```python
from build123d import *

# Parameters (mm, degrees)
F1_DEPTH  = 2
F2_DEPTH  = 10
F3_R      = 4
F4_DEPTH  = 10.001
F3_R_2    = 11
F5_DEPTH  = 8
F6_R      = 4
F7_DEPTH  = 10.001
F6_R_2    = 11
F8_DEPTH  = 8
F10_DEPTH = 8


with BuildPart() as f1:
    # F0 (on Top) → F1 (new body)
    with BuildSketch(Plane.XY):
        with BuildLine():
            ThreePointArc((12, 5), (11.7240041235, 2.4411472664), (10.9087121146, 0))
            Line((10.9087121146, 0), (69.0912878854, 0))
            ThreePointArc((69.0912878854, 0), (68, 5), (69.0912878854, 10))
            Line((69.0912878854, 10), (10.9087121146, 10))
            ThreePointArc((10.9087121146, 10), (11.7240041235, 7.5588527336), (12, 5))
        make_face()
    extrude(amount=F1_DEPTH)

    # F0 (on Top) → F2 (join)
    with BuildSketch(Plane.XY):
        with BuildLine():
            Line((10.9087121146, 0), (0, 0))
            Line((0, 0), (0, 10))
            Line((0, 10), (10.9087121146, 10))
            ThreePointArc((10.9087121146, 10), (-12, 5), (10.9087121146, 0))
        make_face()
        with BuildLine():
            ThreePointArc((69.0912878854, 10), (68, 5), (69.0912878854, 0))
            Line((69.0912878854, 0), (80, 0))
            Line((80, 0), (80, 10))
            Line((80, 10), (69.0912878854, 10))
        make_face()
        with BuildLine():
            Line((80, 0), (69.0912878854, 0))
            ThreePointArc((69.0912878854, 0), (82.5588527336, -6.7240041235), (92, 5))
            ThreePointArc((92, 5), (82.5588527336, 16.7240041235), (69.0912878854, 10))
            Line((69.0912878854, 10), (80, 10))
            Line((80, 10), (80, 0))
        make_face()
        with BuildLine():
            Line((0, 10), (0, 0))
            Line((0, 0), (10.9087121146, 0))
            ThreePointArc((10.9087121146, 0), (11.7240041235, 2.4411472664), (12, 5))
            ThreePointArc((12, 5), (11.7240041235, 7.5588527336), (10.9087121146, 10))
            Line((10.9087121146, 10), (0, 10))
        make_face()
    extrude(amount=F2_DEPTH)

    # F3 (on face) → F4 (cut, through all)
    with BuildSketch(Plane.XY.offset(10)):
        with Locations((0, 5)):
            Circle(F3_R)
    extrude(amount=-F4_DEPTH, mode=Mode.SUBTRACT)

    # F3 (on face) → F5 (cut)
    with BuildSketch(Plane.XY.offset(10)):
        with Locations((0, 5)):
            Circle(F3_R_2)
        with Locations((0, 5)):
            Circle(F3_R, mode=Mode.SUBTRACT)
    extrude(amount=-F5_DEPTH, mode=Mode.SUBTRACT)

    # F6 (on face) → F7 (cut, through all)
    with BuildSketch(Plane.XY.offset(10)):
        with Locations((80, 5)):
            Circle(F6_R)
    extrude(amount=-F7_DEPTH, mode=Mode.SUBTRACT)

    # F6 (on face) → F8 (cut)
    with BuildSketch(Plane.XY.offset(10)):
        with Locations((80, 5)):
            Circle(F6_R_2)
        with Locations((80, 5)):
            Circle(F6_R, mode=Mode.SUBTRACT)
    extrude(amount=-F8_DEPTH, mode=Mode.SUBTRACT)

    # F9 (on face) → F10 (join)
    with BuildSketch(Plane.XY.offset(2)):
        with BuildLine():
            ThreePointArc((10.9087121146, 10), (11.3081338214, 9.0157327447), (11.6189500386, 8))
            Line((11.6189500386, 8), (68.3810499614, 8))
            ThreePointArc((68.3810499614, 8), (68.6918661786, 9.0157327447), (69.0912878854, 10))
            Line((69.0912878854, 10), (10.9087121146, 10))
        make_face()
        with BuildLine():
            ThreePointArc((11.6189500386, 2), (11.3081338214, 0.9842672553), (10.9087121146, 0))
            Line((10.9087121146, 0), (69.0912878854, 0))
            ThreePointArc((69.0912878854, 0), (68.6918661786, 0.9842672553), (68.3810499614, 2))
            Line((68.3810499614, 2), (11.6189500386, 2))
        make_face()
    extrude(amount=F10_DEPTH)


solid = f1.part
```
The listing builds one solid part. Answer for the finished solid, in the listing's coordinates (mm). A direction names the side the tool comes from. Coordinates: 2 decimals unless noted, no trailing zeros. Write each loop counter-clockwise with the first axis right and the second up, starting at its lowest first coordinate (ties: lowest second). Pieces come first, ordered by that corner, then holes.
Q1. Section D-D, the plane x = 18 is taken. Write down the section's boundary in (y, z).
Returned:
outline: (0, 0) - (10, 0) - (10, 10) - (8, 10) - (8, 2) - (2, 2) - (2, 10) - (0, 10) - close
Q2. The mould has two halves that part along X. Classify faces 4 (the flat face through (40, 0, 5)), 5 (the flat face through (0, 0, 2)), 6 (the flat face through (40, 9, 10)): released by +X, released by -X, zero draft, split by the parting line, or undercut.
Returned:
face 4: undercut
face 5: undercut
face 6: zero draft
Q3. Find the intervals of material crossed by line 1 along Y through (x, z) = (0, 7); line 2 along Y through (x, z) = (0, 1.1); line 3 along X through (y, z) = (3.25, 4.25), in increasing order.
Returned:
line 1: y = -7 to -6, 16 to 17
line 2: y = -7 to 1, 9 to 17
line 3: x = -11.87 to -10.86, 10.86 to 11.87, 68.13 to 69.14, 90.86 to 91.87
Q4. Section C-C, the plane y = -1.25 is taken. Write down the section's boundary in (x, z), then the cut area to 3 significant figures.
Returned:
outline: (-10.24, 0) - (10.24, 0) - (10.24, 10) - (9.05, 10) - (9.05, 2) - (-9.05, 2) - (-9.05, 10) - (-10.24, 10) - close; (69.76, 0) - (90.24, 0) - (90.24, 10) - (89.05, 10) - (89.05, 2) - (70.95, 2) - (70.95, 10) - (69.76, 10) - close
area: 120 mm2
Q5. Given P1, Ø5, axis at y = 2, z = 4.5, coming from the -X side; P2, Ø4, axis at y = 14, z = 6.5, coming from the +X side; P3, Ø11, axis at x = -2.5, y = 8, coming from the +Z side, each flat-ended and moving along its own axis, determine where each tip first touches the part or whether it passes through.
Returned:
P1: stops at x = -11.99
P2: stops at x = 89.75
P3: stops at z = 2
Q6. Section A-A, the plane z = 4.25 is taken. Write down the section's boundary in (x, y).
Returned:
outline: (10.91, 0) - (69.09, 0) arc R12 ccw (long way) to (69.09, 10) - (10.91, 10) arc R12 ccw (long way) to start; hole circle Ø22 at (0, 5); hole (11.62, 2) - (68.38, 2) arc R12 cw to (68.38, 8) - (11.62, 8) arc R12 cw to start; hole circle Ø22 at (80, 5)
Q7. Section B-B, the plane x = 0 is taken. Write down the section's boundary in (y, z).
Returned:
outline: (-7, 0) - (1, 0) - (1, 2) - (-6, 2) - (-6, 10) - (-7, 10) - close; (9, 0) - (17, 0) - (17, 10) - (16, 10) - (16, 2) - (9, 2) - close
Q8. Which of the six approach directions +Z, -Z, +X, -X, +Y, -Y give full straight-line access (tool end or side, diameter ignored) to faces 1 (the cylindrical face through (76, 5, 1)), 2 (the flat face through (40, 10, 5)), 3 (the cylindrical face through (69, 5, 6))?
Returned:
face 1: +Z, -Z
face 2: +Z, -Z, +Y
face 3: +Z
